Print and shaded views of the part. All mm, measured from the part's lowest x, y and z. A direction names the side the tool comes from. Round coordinates to 2 decimals unless told otherwise and drop trailing zeros. Loops run counter-clockwise (first coordinate to the right, second up) from the corner with the lowest first, then second, coordinate; pieces in that order, holes last. Notation, with made-up numbers: (-17.75, -16) -> (28.25, -16) arc R8 ccw to (28.25, -1) -> close; hole circle Ø8 at (10.25, -12). An arc over 180 degrees is marked (long way). Use a Markdown table: item, result.
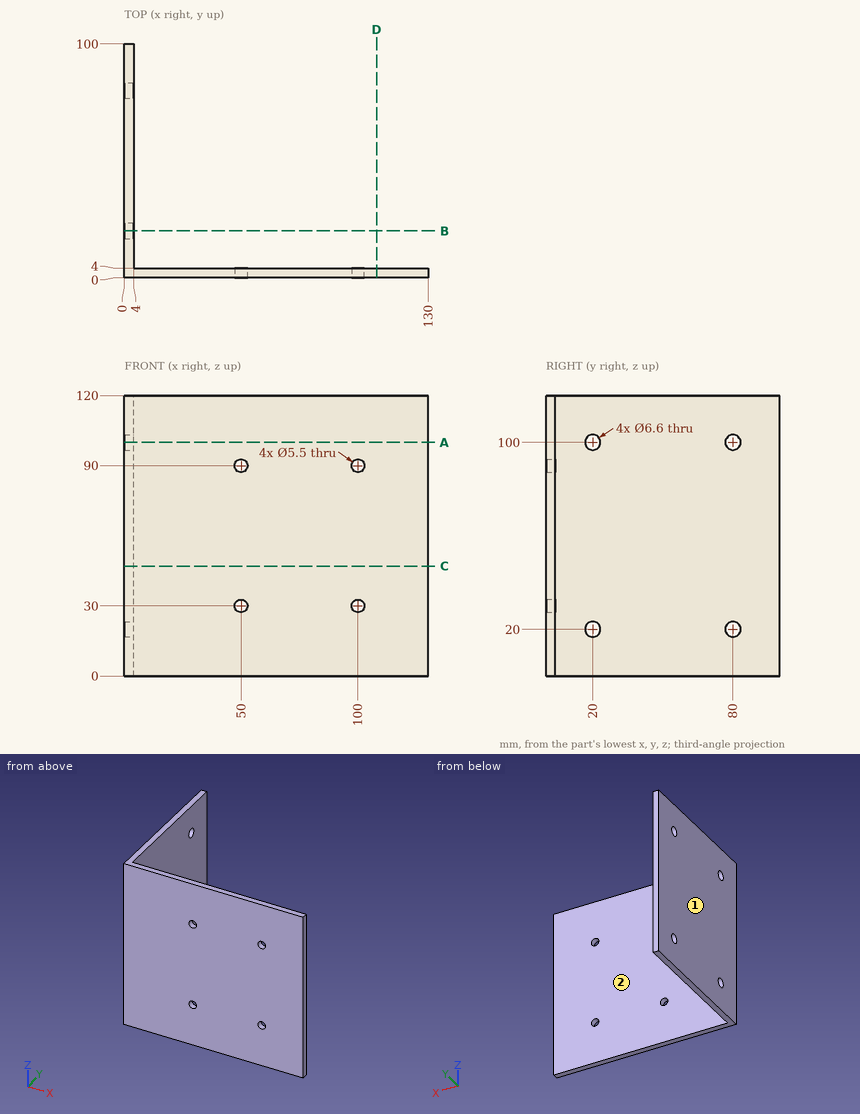
Q1. Band-saw the part on D-D, the plane x = 108. Give the cut face in (y, z).
Results list:
| item | result |
|---|---|
| outline | (0, 0) -> (4, 0) -> (4, 120) -> (0, 120) -> close |
Q2. Tool access for the marked faces 1 and 2: list every direction of +Z, -Z, +X, -X, +Y, -Y with a clear straight run to the whole face (end or side of a thin tool).
Results list:
| item | result |
|---|---|
| face 1 | +Z, -Z, -X, +Y, -Y |
| face 2 | +Z, -Z, +X, +Y |
Q3. Flat gauge pins, fed straight in: pin 1 (10.5 mm diameter, centred on y = 20, z = 100, fed in from +X); pin 2 (9 mm diameter, centred on x = 50, z = 30, fed in from +Y). Where does each tip first touch, or does it go through?
Results list:
| item | result |
|---|---|
| pin 1 | stops at x = 4 |
| pin 2 | stops at y = 4 |
Q4. Band-saw the part on C-C, the plane z = 47. Give the cut face in (x, y).
Results list:
| item | result |
|---|---|
| outline | (0, 0) -> (130, 0) -> (130, 4) -> (4, 4) -> (4, 100) -> (0, 100) -> close |
Q5. Drill centre lines: L1, parallel to Z at x = 1.7, y = 80; L2, parallel to Z at x = 50, y = 2.6; L3, parallel to Y at x = 87, z = 32.5. Where is each one in solid material? Low to high. Write a range as from..to.
Results list:
| item | result |
|---|---|
| L1 | z = 0..16.7, 23.3..96.7, 103.3..120 |
| L2 | z = 0..27.25, 32.75..87.25, 92.75..120 |
| L3 | y = 0..4 |
Q6. Band-saw the part on B-B, the plane y = 20. Give the cut face in (x, z), plus the area to 3 significant figures.
Results list:
| item | result |
|---|---|
| outline | (0, 0) -> (4, 0) -> (4, 16.7) -> (0, 16.7) -> close; (0, 23.3) -> (4, 23.3) -> (4, 96.7) -> (0, 96.7) -> close; (0, 103.3) -> (4, 103.3) -> (4, 120) -> (0, 120) -> close |
| area | 427 mm² |
Q7. Band-saw the part on A-A, the plane z = 100. Give the cut face in (x, y), plus the area to 3 significant figures.
Results list:
| item | result |
|---|---|
| outline | (0, 0) -> (130, 0) -> (130, 4) -> (4, 4) -> (4, 16.7) -> (0, 16.7) -> close; (0, 23.3) -> (4, 23.3) -> (4, 76.7) -> (0, 76.7) -> close; (0, 83.3) -> (4, 83.3) -> (4, 100) -> (0, 100) -> close |
| area | 851 mm² |
